from build123d import *

# Parameters (mm, degrees)
BOSS_EXTRUDE1_DEPTH     = 3
M4_CLEARANCE_HOLE1_D    = 4.5
SKETCH5_R               = 2
CUT_EXTRUDE1_DEPTH      = 20
SKETCH8_R               = 3
CUT_EXTRUDE3_DEPTH      = 4.4
CUT_EXTRUDE4_DEPTH      = 25.596747752
BOSS_EXTRUDE2_DEPTH     = 1.5
FILLET1_R               = 1
CUT_EXTRUDE2_DEPTH      = 25.274472342
CUT_EXTRUDE2_DEPTH_BACK = 25.274472342
SKETCH7_R               = 0.75
BOSS_EXTRUDE3_START     = -6
SKETCH10_R              = 1.5
BOSS_EXTRUDE3_DEPTH     = 6
FILLET3_R               = 2


with BuildPart() as part:
    # Sketch2 → Boss-Extrude1 (new, symmetric)
    with BuildSketch(Plane.XY):
        with BuildLine():
            Line((13, 0), (13, -20))
            Line((13, -20), (7, -20))
            Line((7, -20), (7, -10.95445115))
            ThreePointArc((7, -10.95445115), (-11.401754251, 6.244997998), (13, 0))
        make_face()
    extrude(amount=BOSS_EXTRUDE1_DEPTH, both=True)

    # M4 Clearance Hole1 (through all)
    with Locations(Plane.XY.offset(3)):
        with Locations((0, 0)):
            Hole(M4_CLEARANCE_HOLE1_D / 2)

    # Sketch5 → Cut-Extrude1 (cut)
    with BuildSketch(Plane.XZ.offset(20)):
        with Locations(Location((10, 0, 0), (0, 0, 270))):
            Circle(SKETCH5_R)
    extrude(amount=-CUT_EXTRUDE1_DEPTH, mode=Mode.SUBTRACT)

    # Sketch8 → Cut-Extrude3 (cut)
    with BuildSketch(Plane.XY.offset(-3)):
        with Locations((-6.894399988, 5.785088487)):
            Circle(SKETCH8_R)
    extrude(amount=CUT_EXTRUDE3_DEPTH, mode=Mode.SUBTRACT)

    # Sketch9 → Cut-Extrude4 (cut, through all)
    with BuildSketch(Plane.XY.offset(3)):
        with BuildLine():
            Line((13, 0), (7.25, 0))
            ThreePointArc((7.25, 0), (4.738095767, 5.487526629), (-1.057020278, 7.172531501))
            ThreePointArc((-1.057020278, 7.172531501), (-2.732190546, 10.106663728), (-5.727165906, 11.670457176))
            ThreePointArc((-5.727165906, 11.670457176), (6.875567003, 11.03297686), (13, 0))
        make_face()
    extrude(amount=-CUT_EXTRUDE4_DEPTH, mode=Mode.SUBTRACT)

    # Sketch6 → Boss-Extrude2 (add, symmetric)
    with BuildSketch(Plane.XY):
        with BuildLine():
            Line((13, 1.5), (13, 0))
            Line((13, 0), (7.25, 0))
            ThreePointArc((7.25, 0), (7.085685326, 1.534784498), (6.600189391, 3))
            Line((6.600189391, 3), (11.5, 3))
            ThreePointArc((11.5, 3), (12.560660172, 2.560660172), (13, 1.5))
        make_face()
    extrude(amount=BOSS_EXTRUDE2_DEPTH, both=True)

    # Fillet1
    fillet1_edges = [part.edges().sort_by_distance(p)[0] for p in [
        (-5.727165906, 11.670457176, 0),
        (7.25, 0, -2.25),
        (-1.057020278, 7.172531501, 0),
        (7.25, 0, 2.25),
        (13, 0, -2.25),
        (13, 0, 2.25),
    ]]
    fillet(fillet1_edges, radius=FILLET1_R)

    # Sketch7 → Cut-Extrude2 (cut, two sides: drawn at the far end of the back side and taken through both)
    with BuildSketch(Plane.XY.offset(1.5).offset(-CUT_EXTRUDE2_DEPTH_BACK)):
        with Locations((11.5, 1.5)):
            Circle(SKETCH7_R)
    extrude(amount=CUT_EXTRUDE2_DEPTH + CUT_EXTRUDE2_DEPTH_BACK, mode=Mode.SUBTRACT)

    # Sketch10 → Boss-Extrude3 (add)
    with BuildSketch(Plane(origin=(0, 0, -3), x_dir=(-1, 0, 0), z_dir=(0, 0, -1)).offset(BOSS_EXTRUDE3_START)):
        with BuildLine():
            Line((-7, -10.95445115), (-7, -20))
            Line((-7, -20), (-1.5, -20))
            Line((-1.5, -20), (-1.5, -12.91317157))
            ThreePointArc((-1.5, -12.91317157), (-4.361381252, -12.246564971), (-7, -10.95445115))
        make_face()
        with Locations((-4.6, -16.5)):
            Circle(SKETCH10_R, mode=Mode.SUBTRACT)
    extrude(amount=BOSS_EXTRUDE3_DEPTH)

    # Fillet3
    fillet3_edges = [part.edges().sort_by_distance(p)[0] for p in [
        (1.5, -12.91317157, 0),
        (1.5, -20, 0),
    ]]
    fillet(fillet3_edges, radius=FILLET3_R)


solid = part.part
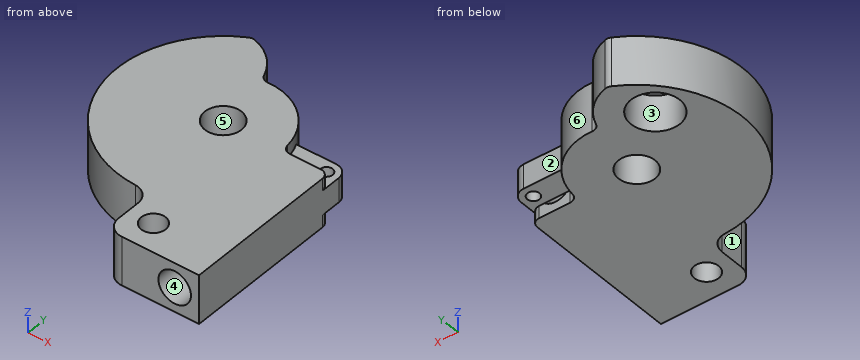
Input: part model. Units: mm. Frame: model coordinates. Face numbers are marked on the shaded views. A direction names the side the tool comes from. Give positions to 0.01 mm unless a question says otherwise; leave off trailing zeros. Order: outer loops, then holes, each group sorted by start corner. A loop starts at its lowest first (then second) coordinate and runs counter-clockwise, first axis right, second up. Notation, with made-up numbers: (5.5, 4) - (22.5, 4) arc R38 cw to (22.5, 42) - close; hole circle Ø2 at (7.25, -2). An arc over 180 degrees is marked (long way). Write each question's results on one line, items separated by ' | '.
Item 1: Section D-D (z = 2.5). Give the number of separate pieces and of enclosed holes in the cut face, and give its area (3 significant figures).
A:
separate pieces: 1 | enclosed holes: 2 | area: 517 mm^2
Item 2: Section C-C (y = -9). Return loops of the section in (x, z).
A:
outline: (-9.38, -3) - (13, -3) - (13, 3) - (-9.38, 3) - close; hole circle Ø4 at (10, 0)
Item 3: Material intervals for line 1 along X through (y, z) = (-9, 1.5); line 2 along Y through (x, z) = (4.6, 0); line 3 along Y through (x, z) = (4.25, -2), sorted ascending.
A:
line 1: x = -9.38 to 8.68, 11.32 to 13 | line 2: y = -20 to -18, -15 to 5.6 | line 3: y = -20 to -17.96, -15.04 to 5.87
Item 4: Section B-B (x = 5.75). Return loops of the section in (y, z).
A:
outline: (-20, -3) - (-17.46, -3) - (-17.46, 3) - (-20, 3) - close; (-15.54, -3) - (4.42, -3) - (4.42, 3) - (-15.54, 3) - close
Item 5: Draft query along Y for the marked faces 4, 5 and 6. Return one class per face: released by +Y, released by -Y, zero draft, split by the parting line, or undercut.
A:
face 4: zero draft | face 5: undercut | face 6: released by +Y
Item 6: Contact query for flat-ended pins moving along their axis: pin 1 Ø0.8 at (x, z) = (9.5, 2.5) entering from +Y; pin 2 Ø2.5 at (x, z) = (10, -0.5) entering from -Y; pin 3 Ø4 at (x, y) = (9, 3) entering from -Z. Output: stop coordinate, or through.
A:
pin 1: stops at y = 0 | pin 2: stops at y = 0 | pin 3: stops at z = -1.5
Item 7: Section A-A (x = 10). Return loops of the section in (y, z), and give its area (3 significant figures).
A:
outline: (-20, -3) - (0, -3) - (0, -2) - (-20, -2) - close; (-20, 2) - (0, 2) - (0, 3) - (-20, 3) - close; (0, -1.5) - (3, -1.5) - (3, 1.5) - (0, 1.5) - close | area: 49.0 mm^2
Item 8: Access query for the marked faces 1, 2 and 3. Directions: +Z, -Z, +X, -X, +Y, -Y. A direction counts if a zero-diameter tool reaches every point of the face in a straight line with its end or side. Return the directions, or none.
A:
face 1: +Z, -Z, -X, -Y | face 2: +Z, -Z, +X, +Y | face 3: -Z
